from build123d import *

# Parameters (mm, degrees)
ESTRUSIONE_ESTRUSIONE1_DEPTH = 1.6


with BuildPart() as part:
    # bordo3 → Estrusione-Estrusione1 (new body)
    with BuildSketch(Plane.XY):
        with BuildLine():
            Line((175.787012069, 105.00274093), (192.58131235, 105.882892913))
            ThreePointArc((192.58131235, 105.882892913), (198.506836606, 103.696851603), (201, 97.893856635))
            Line((201, 97.893856635), (201, -7.091597346))
            ThreePointArc((201, -7.091597346), (198.656854249, -12.748451596), (193, -15.091597346))
            Line((193, -15.091597346), (117.750790543, -15.091597346))
            ThreePointArc((117.750790543, -15.091597346), (116.336576981, -14.505810909), (115.750790543, -13.091597346))
            Line((115.750790543, -13.091597346), (115.750790543, -12.967534141))
            ThreePointArc((115.750790543, -12.967534141), (115.127499694, -11.516785399), (113.64611863, -10.970275071))
            Line((113.64611863, -10.970275071), (0.928841556, -16.877537249))
            ThreePointArc((0.928841556, -16.877537249), (-0.145141858, -16.910699844), (-1.219558299, -16.897682863))
            Line((-1.219558299, -16.897682863), (-151.023233988, -11.861429997))
            ThreePointArc((-151.023233988, -11.861429997), (-156.505538032, -9.426954116), (-158.754433684, -3.865947122))
            Line((-158.754433684, -3.865947122), (-158.754433684, 95.67986032))
            ThreePointArc((-158.754433684, 95.67986032), (-156.26127029, 101.482855288), (-150.335746034, 103.668896598))
            Line((-150.335746034, 103.668896598), (-140.339889089, 103.145035933))
            ThreePointArc((-140.339889089, 103.145035933), (-134.414364833, 105.331077243), (-131.921201439, 111.134072211))
            Line((-131.921201439, 111.134072211), (-131.921201439, 118.187089821))
            ThreePointArc((-131.921201439, 118.187089821), (-129.578055688, 123.843944071), (-123.921201439, 126.187089821))
            Line((-123.921201439, 126.187089821), (-86.871201439, 126.187089821))
            ThreePointArc((-86.871201439, 126.187089821), (-81.214347189, 123.843944071), (-78.871201439, 118.187089821))
            Line((-78.871201439, 118.187089821), (-78.871201439, 107.515315052))
            ThreePointArc((-78.871201439, 107.515315052), (-76.674196407, 102.008478446), (-71.289889089, 99.526278774))
            Line((-71.289889089, 99.526278774), (-2.104671912, 95.900435182))
            ThreePointArc((-2.104671912, 95.900435182), (-0.623290849, 96.44694551), (0, 97.897694252))
            Line((0, 97.897694252), (0, 100.897694252))
            ThreePointArc((0, 100.897694252), (0.549251258, 102.274403403), (1.895328088, 102.894953321))
            Line((1.895328088, 102.894953321), (97.91868765, 107.927324355))
            ThreePointArc((97.91868765, 107.927324355), (99.939463207, 107.499136975), (101.477166344, 106.11988089))
            Line((101.477166344, 106.11988089), (102.479467612, 104.76578913))
            ThreePointArc((102.479467612, 104.76578913), (105.496696561, 102.289889033), (109.326285673, 101.536231916))
            Line((109.326285673, 101.536231916), (175.787012069, 105.00274093))
        make_face()
        with BuildLine():
            Line((122.250790543, -7.091597346), (122.250790543, 10.907402654))
            ThreePointArc((122.250790543, 10.907402654), (122.690130371, 11.968062825), (123.750790543, 12.407402654))
            Line((123.750790543, 12.407402654), (139.800790543, 12.407402654))
            ThreePointArc((139.800790543, 12.407402654), (140.861450715, 12.846742482), (141.300790543, 13.907402654))
            Line((141.300790543, 13.907402654), (141.300790543, 29.957402654))
            ThreePointArc((141.300790543, 29.957402654), (141.740130371, 31.018062825), (142.800790543, 31.457402654))
            Line((142.800790543, 31.457402654), (160.800790543, 31.457402654))
            ThreePointArc((160.800790543, 31.457402654), (161.861450715, 31.018062825), (162.300790543, 29.957402654))
            Line((162.300790543, 29.957402654), (162.300790543, 13.907402654))
            ThreePointArc((162.300790543, 13.907402654), (162.740130371, 12.846742482), (163.800790543, 12.407402654))
            Line((163.800790543, 12.407402654), (179.850790543, 12.407402654))
            ThreePointArc((179.850790543, 12.407402654), (180.911450715, 11.968062825), (181.350790543, 10.907402654))
            Line((181.350790543, 10.907402654), (181.350790543, -7.091597346))
            ThreePointArc((181.350790543, -7.091597346), (180.911450715, -8.152257518), (179.850790543, -8.591597346))
            Line((179.850790543, -8.591597346), (123.750790543, -8.591597346))
            ThreePointArc((123.750790543, -8.591597346), (122.690130371, -8.152257518), (122.250790543, -7.091597346))
        make_face(mode=Mode.SUBTRACT)
        with BuildLine():
            Line((5.921496066, 89.591546211), (141.282050751, 96.685492285))
            Line((141.282050751, 96.685492285), (177.852024899, 96.679778694))
            ThreePointArc((177.852024899, 96.679778694), (178.912533569, 96.240356024), (179.351790543, 95.179778713))
            Line((179.351790543, 95.179778713), (179.351790543, 77.179309781))
            ThreePointArc((179.351790543, 77.179309781), (179.791047517, 76.11873247), (180.851556187, 75.6793098))
            Line((180.851556187, 75.6793098), (193.000234356, 75.677411724))
            ThreePointArc((193.000234356, 75.677411724), (194.060743026, 75.237989054), (194.5, 74.177411743))
            Line((194.5, 74.177411743), (194.5, 16.9505))
            ThreePointArc((194.5, 16.9505), (194.060660172, 15.889839828), (193, 15.4505))
            Line((193, 15.4505), (175, 15.4505))
            ThreePointArc((175, 15.4505), (173.939339828, 15.889839828), (173.5, 16.9505))
            Line((173.5, 16.9505), (173.5, 36.605240872))
            ThreePointArc((173.5, 36.605240872), (173.060660172, 37.665901044), (172, 38.105240872))
            Line((172, 38.105240872), (152.727925239, 38.105240872))
            Line((152.727925239, 38.105240872), (129.729835534, 36.899962063))
            ThreePointArc((129.729835534, 36.899962063), (128.69362223, 36.405713671), (128.310395167, 35.323513827))
            Line((128.310395167, 35.323513827), (129.150382031, 19.295609657))
            ThreePointArc((129.150382031, 19.295609657), (128.767154967, 18.213409813), (127.730941663, 17.71916142))
            Line((127.730941663, 17.71916142), (105.950202838, 16.577681267))
            ThreePointArc((105.950202838, 16.577681267), (104.913989534, 16.083432875), (104.53076247, 15.001233031))
            Line((104.53076247, 15.001233031), (105.60810129, -5.555616249))
            ThreePointArc((105.60810129, -5.555616249), (105.216302409, -6.647255074), (104.163185056, -7.133182565))
            Line((104.163185056, -7.133182565), (9, -10.4995))
            Line((9, -10.4995), (-9, -10.4995))
            Line((-9, -10.4995), (-113.037709318, -6.819253752))
            Line((-113.037709318, -6.819253752), (-128.763233684, -6.819253752))
            ThreePointArc((-128.763233684, -6.819253752), (-129.823893856, -6.379913923), (-130.263233684, -5.319253752))
            Line((-130.263233684, -5.319253752), (-130.263233684, 3.650335982))
            ThreePointArc((-130.263233684, 3.650335982), (-130.702573513, 4.710996153), (-131.763233684, 5.150335982))
            Line((-131.763233684, 5.150335982), (-150.754433684, 5.150335982))
            ThreePointArc((-150.754433684, 5.150335982), (-151.815093856, 5.58967581), (-152.254433684, 6.650335982))
            Line((-152.254433684, 6.650335982), (-152.254433684, 24.649335982))
            ThreePointArc((-152.254433684, 24.649335982), (-151.815093856, 25.709996153), (-150.754433684, 26.149335982))
            Line((-150.754433684, 26.149335982), (-141.025733684, 26.149335982))
            ThreePointArc((-141.025733684, 26.149335982), (-139.965073513, 26.58867581), (-139.525733684, 27.649335982))
            Line((-139.525733684, 27.649335982), (-139.525733684, 55.176535982))
            ThreePointArc((-139.525733684, 55.176535982), (-139.086393856, 56.237196153), (-138.025733684, 56.676535982))
            Line((-138.025733684, 56.676535982), (-136.394433684, 56.676535982))
            ThreePointArc((-136.394433684, 56.676535982), (-135.333773513, 57.11587581), (-134.894433684, 58.176535982))
            Line((-134.894433684, 58.176535982), (-134.894433684, 78.277535982))
            ThreePointArc((-134.894433684, 78.277535982), (-135.333773513, 79.338196153), (-136.394433684, 79.777535982))
            Line((-136.394433684, 79.777535982), (-148.181933684, 79.777535982))
            ThreePointArc((-148.181933684, 79.777535982), (-149.242593856, 80.21687581), (-149.681933684, 81.277535982))
            Line((-149.681933684, 81.277535982), (-149.681933684, 99.276535982))
            ThreePointArc((-149.681933684, 99.276535982), (-149.242593856, 100.337196153), (-148.181933684, 100.776535982))
            Line((-148.181933684, 100.776535982), (-126.921201439, 100.776535982))
            ThreePointArc((-126.921201439, 100.776535982), (-125.860541267, 101.21587581), (-125.421201439, 102.276535982))
            Line((-125.421201439, 102.276535982), (-125.421201439, 118.187089821))
            ThreePointArc((-125.421201439, 118.187089821), (-124.981861611, 119.247749993), (-123.921201439, 119.687089821))
            Line((-123.921201439, 119.687089821), (-86.871201439, 119.687089821))
            ThreePointArc((-86.871201439, 119.687089821), (-85.810541267, 119.247749993), (-85.371201439, 118.187089821))
            Line((-85.371201439, 118.187089821), (-85.371201439, 95.178775684))
            ThreePointArc((-85.371201439, 95.178775684), (-84.959262995, 94.146243821), (-83.949705373, 93.680831382))
            Line((-83.949705373, 93.680831382), (-13.061697239, 89.965748298))
            Line((-13.061697239, 89.965748298), (-5.921496066, 89.591546211))
            ThreePointArc((-5.921496066, 89.591546211), (-4.885282762, 89.097297818), (-4.502055698, 88.015097975))
            Line((-4.502055698, 88.015097975), (-8.481750162, 12.078003934))
            ThreePointArc((-8.481750162, 12.078003934), (-8.071867416, 10.966968136), (-6.98380586, 10.4995))
            Line((-6.98380586, 10.4995), (6.98380586, 10.4995))
            ThreePointArc((6.98380586, 10.4995), (8.071867416, 10.966968136), (8.481750162, 12.078003934))
            Line((8.481750162, 12.078003934), (4.502055698, 88.015097974))
            ThreePointArc((4.502055698, 88.015097974), (4.885282762, 89.097297818), (5.921496066, 89.591546211))
        make_face(mode=Mode.SUBTRACT)
    extrude(amount=ESTRUSIONE_ESTRUSIONE1_DEPTH)


solid = part.part
Check sheet for the modelled part. Datum: model origin and axes. Units: mm. A direction names the side the tool comes from. Give positions to 0.01 mm unless a question says otherwise; leave off trailing zeros. Loops run counter-clockwise (first coordinate to the right, second up) from the corner with the lowest first, then second, coordinate; pieces in that order, holes last. Notation, with made-up numbers: M 77,-11.75 L 94,-11.75 A20 ccw 94,6.25 Z; hole C 75,21 d8. An arc over 180 degrees is marked long. Answer as a JSON object with one key per item and string values. Group by question number.
Q1. Cross-section at C-C on z = 0.6. Give the number of separate pieces and of enclosed holes in the cut face, then the cut area to 3 significant figures.
Q2. Material ranges on line 1 along Y through (x, z) = (167.5, 1.3); line 2 along X through (y, z) = (88, 0.3); line 3 along X through (y, z) = (19, 0.6), recorded low to high. Write a range as [from, to].
Q3. Cross-section at D-D on x = 41. Record the cut outline in (y, z), then the cut area to 3 significant figures.
Q4. Cross-section at B-B on y = 64. Record the cut outline in (x, z).
Q5. Access from +Z, -Z, +X, -X, +Y, -Y to the whole of each face (thin tool, end or side, straight path). Record for faces 4 (the cylindrical face through (-76.73, 102.07, 0.79)), 5 (the flat face through (35, 92, 0)), 6 (the flat face through (58.077, -13.883, 0.789)).
Q6. Cross-section at A-A on x = 85. Record the cut outline in (y, z).
Q7. Release check for a two-part mould opening along Y. For faces 1 (the flat face through (35, 92, 1.6)), 2 (the flat face through (72.65, 93.09, 0.79)), 3 (the cylindrical face through (-156.327, 101.42, 0.789)) record: released by +Y, released by -Y, zero draft, split by the parting line, or undercut.
Q8. Go/stop test with flat-tipped pins: P1, Ø0.5, axis at y = 116, z = 0.5, coming from the -X side; P2, Ø0.8, axis at x = 185.5, z = 1, coming from the -Y side; P3, Ø0.8, axis at x = 163, z = 1, coming from the +Y side. Record where each tip stops, or that it passes through.
Evaluation:
{
 "1": {"separate pieces": "1", "enclosed holes": "2", "area": "10,800 mm2"},
 "2": {"line 1": "y = [-15.09, -8.59], [12.41, 38.11], [96.68, 104.57]", "line 2": "x = [-158.75, -149.68], [-4.5, 4.5], [179.35, 201]", "line 3": "x = [-158.75, -152.25], [-8.12, 8.12], [129.14, 141.3], [162.3, 173.5], [194.5, 201]"},
 "3": {"outline": "M -14.78,0 L -9.37,0 L -9.37,1.6 L -14.78,1.6 Z; M 91.43,0 L 104.94,0 L 104.94,1.6 L 91.43,1.6 Z", "area": "30.3 mm2"},
 "4": {"outline": "M -158.75,0 L -134.89,0 L -134.89,1.6 L -158.75,1.6 Z; M -5.76,0 L 5.76,0 L 5.76,1.6 L -5.76,1.6 Z; M 194.5,0 L 201,0 L 201,1.6 L 194.5,1.6 Z"},
 "5": {"face 4": "+Z, -Z, +Y", "face 5": "-Z, +X, -X, +Y, -Y", "face 6": "+Z, -Z, -Y"},
 "6": {"outline": "M -12.47,0 L -7.81,0 L -7.81,1.6 L -12.47,1.6 Z; M 93.74,0 L 107.25,0 L 107.25,1.6 L 93.74,1.6 Z"},
 "7": {"face 1": "zero draft", "face 2": "undercut", "face 3": "released by +Y"},
 "8": {"P1": "stops at x = -131.92", "P2": "stops at y = -15.09", "P3": "stops at y = 104.36"}
}
